Geometry check sheet. Reference: the model listing, model coordinates, mm. A direction names the side the tool comes from. Give positions to 0.01 mm unless a question says otherwise; leave off trailing zeros. Write each loop counter-clockwise with the first axis right and the second up, starting at its lowest first coordinate (ties: lowest second). Pieces come first, ordered by that corner, then holes. Notation, with made-up numbers: (-5.5, 39) - (51.5, 39) arc R25 ccw to (51.5, 72) - close; hole circle Ø8 at (16, 20). An arc over 180 degrees is marked (long way). Use a Markdown table: item, result.
```python
from build123d import *

# Parameters (mm, degrees)
F0_R     = 14.5472790553
F1_DEPTH = 3.175
F2_DEPTH = 5.715


with BuildPart() as f1:
    # F0 (on Top) → F1 (new body)
    with BuildSketch(Plane.XY):
        with BuildLine():
            add(Edge.make_bspline(
                [(-17.3302307441, -18.9114744135), (-12.7840517895, -39.3035737815), (-3.2940015008, -39.2257868182)],
                knots=[5.1919648614, 5.1919648614, 5.1919648614, 6.2831853072, 6.2831853072, 6.2831853072], degree=2, weights=[1, 0.854810781, 1]))
            add(Edge.make_bspline(
                [(-3.2940015008, -39.2257868182), (6.123923112, -39.1485910465), (10.3601545856, -18.9114744135)],
                knots=[0, 0, 0, 1.0844638725, 1.0844638725, 1.0844638725], degree=2, weights=[1, 0.8565590272, 1]))
            add(Edge.make_bspline(
                [(10.3601545856, -18.9114744135), (12.1044870422, -10.5785351982), (12.0273641605, -1.1695031996)],
                knots=[1.0844638725, 1.0844638725, 1.0844638725, 1.5707963268, 1.5707963268, 1.5707963268], degree=2, weights=[1, 0.9705804868, 1]))
            add(Edge.make_bspline(
                [(12.0273641605, -1.1695031996), (11.88861373, 15.7581220548), (6.6027932897, 27.0196823223)],
                knots=[1.5707963268, 1.5707963268, 1.5707963268, 2.4103546369, 2.4103546369, 2.4103546369], degree=2, weights=[1, 0.9131789699, 1]))
            ThreePointArc((6.6027932897, 27.0196823223), (-3.7977289586, 22.4602209118), (-14.2062252861, 27.0014493351))
            add(Edge.make_bspline(
                [(-14.2062252861, 27.0014493351), (-19.3770142282, 15.6392708689), (-19.2371374573, -1.4257685052)],
                knots=[3.8667963971, 3.8667963971, 3.8667963971, 4.7123889804, 4.7123889804, 4.7123889804], degree=2, weights=[1, 0.9119451548, 1]))
            add(Edge.make_bspline(
                [(-19.2371374573, -1.4257685052), (-19.1611285396, -10.6988963006), (-17.3302307441, -18.9114744135)],
                knots=[4.7123889804, 4.7123889804, 4.7123889804, 5.1919648614, 5.1919648614, 5.1919648614], degree=2, weights=[1, 0.9713883601, 1]))
        make_face()
        with Locations((-3.6048866484, -1.2976358524)):
            Circle(F0_R, mode=Mode.SUBTRACT)
    extrude(amount=F1_DEPTH)

    # F0 (on Top) → F2 (join)
    with BuildSketch(Plane.XY):
        with BuildLine():
            add(Edge.make_bspline(
                [(-17.3302307441, -18.9114744135), (-12.7840517895, -39.3035737815), (-3.2940015008, -39.2257868182)],
                knots=[5.1919648614, 5.1919648614, 5.1919648614, 6.2831853072, 6.2831853072, 6.2831853072], degree=2, weights=[1, 0.854810781, 1]))
            add(Edge.make_bspline(
                [(-3.2940015008, -39.2257868182), (6.123923112, -39.1485910465), (10.3601545856, -18.9114744135)],
                knots=[0, 0, 0, 1.0844638725, 1.0844638725, 1.0844638725], degree=2, weights=[1, 0.8565590272, 1]))
            add(Edge.make_bspline(
                [(10.3601545856, -18.9114744135), (12.1044870422, -10.5785351982), (12.0273641605, -1.1695031996)],
                knots=[1.0844638725, 1.0844638725, 1.0844638725, 1.5707963268, 1.5707963268, 1.5707963268], degree=2, weights=[1, 0.9705804868, 1]))
            add(Edge.make_bspline(
                [(12.0273641605, -1.1695031996), (11.88861373, 15.7581220548), (6.6027932897, 27.0196823223)],
                knots=[1.5707963268, 1.5707963268, 1.5707963268, 2.4103546369, 2.4103546369, 2.4103546369], degree=2, weights=[1, 0.9131789699, 1]))
            ThreePointArc((6.6027932897, 27.0196823223), (-3.7977289586, 22.4602209118), (-14.2062252861, 27.0014493351))
            add(Edge.make_bspline(
                [(-14.2062252861, 27.0014493351), (-19.3770142282, 15.6392708689), (-19.2371374573, -1.4257685052)],
                knots=[3.8667963971, 3.8667963971, 3.8667963971, 4.7123889804, 4.7123889804, 4.7123889804], degree=2, weights=[1, 0.9119451548, 1]))
            add(Edge.make_bspline(
                [(-19.2371374573, -1.4257685052), (-19.1611285396, -10.6988963006), (-17.3302307441, -18.9114744135)],
                knots=[4.7123889804, 4.7123889804, 4.7123889804, 5.1919648614, 5.1919648614, 5.1919648614], degree=2, weights=[1, 0.9713883601, 1]))
        make_face()
        with Locations((-3.6048866484, -1.2976358524)):
            Circle(F0_R, mode=Mode.SUBTRACT)
        with BuildLine():
            add(Edge.make_bspline(
                [(10.3601545856, -18.9114744135), (12.1044870422, -10.5785351982), (12.0273641605, -1.1695031996)],
                knots=[1.0844638725, 1.0844638725, 1.0844638725, 1.5707963268, 1.5707963268, 1.5707963268], degree=2, weights=[1, 0.9705804868, 1]))
            Line((10.3601545856, -18.9114744135), (10.3601545856, -45.1457377323))
            Line((10.3601545856, -45.1457377323), (23.0601545856, -45.1457377323))
            Line((23.0601545856, -45.1457377323), (12.0273641605, -1.1695031996))
        make_face()
        with BuildLine():
            Line((-17.3302307441, -45.1457377323), (-17.3302307441, -18.9114744135))
            add(Edge.make_bspline(
                [(-19.2371374573, -1.4257685052), (-19.1611285396, -10.6988963006), (-17.3302307441, -18.9114744135)],
                knots=[4.7123889804, 4.7123889804, 4.7123889804, 5.1919648614, 5.1919648614, 5.1919648614], degree=2, weights=[1, 0.9713883601, 1]))
            Line((-19.2371374573, -1.4257685052), (-30.0302307441, -45.1457377323))
            Line((-30.0302307441, -45.1457377323), (-17.3302307441, -45.1457377323))
        make_face()
        with BuildLine():
            Line((23.0601545856, -45.1457377323), (10.3601545856, -45.1457377323))
            ThreePointArc((10.3601545856, -45.1457377323), (16.7101545856, -53.2856193183), (23.0601545856, -45.1457377323))
        make_face()
        with BuildLine():
            ThreePointArc((-30.0302307441, -45.1457377323), (-23.6802307441, -53.2539903225), (-17.3302307441, -45.1457377323))
            Line((-17.3302307441, -45.1457377323), (-30.0302307441, -45.1457377323))
        make_face()
        with BuildLine():
            ThreePointArc((-14.2062252861, 27.0014493351), (-3.7977289586, 22.4602209118), (6.6027932897, 27.0196823223))
            add(Edge.make_bspline(
                [(6.6027932897, 27.0196823223), (2.1602516195, 36.4846180548), (-3.704532498, 36.6287842303)],
                knots=[2.4103546369, 2.4103546369, 2.4103546369, 3.1280810135, 3.1280810135, 3.1280810135], degree=2, weights=[1, 0.9362966883, 1]))
            ThreePointArc((-3.704532498, 36.6287842303), (-3.8110105262, 36.5248919189), (-3.9157717959, 36.6305151135))
            add(Edge.make_bspline(
                [(-3.9157717959, 36.6305151135), (-9.8462768465, 36.5819046252), (-14.2062252861, 27.0014493351)],
                knots=[3.1415926536, 3.1415926536, 3.1415926536, 3.8667963971, 3.8667963971, 3.8667963971], degree=2, weights=[1, 0.9349770844, 1]))
        make_face()
        with BuildLine():
            add(Edge.make_bspline(
                [(6.6027932897, 27.0196823223), (2.1602516195, 36.4846180548), (-3.704532498, 36.6287842303)],
                knots=[2.4103546369, 2.4103546369, 2.4103546369, 3.1280810135, 3.1280810135, 3.1280810135], degree=2, weights=[1, 0.9362966883, 1]))
            ThreePointArc((6.6027932897, 27.0196823223), (9.387427608, 31.4709155445), (10.3601545856, 36.6305151135))
            ThreePointArc((10.3601545856, 36.6305151135), (9.3748938948, 41.8220601436), (6.55612214, 46.2916691))
            ThreePointArc((6.55612214, 46.2916691), (-3.8101450556, 50.8008147547), (-14.1764122512, 46.2916691))
            ThreePointArc((-14.1764122512, 46.2916691), (-16.9951840059, 41.8220601436), (-17.9804446968, 36.6305151135))
            ThreePointArc((-17.9804446968, 36.6305151135), (-17.0031917826, 31.459353737), (-14.2062252861, 27.0014493351))
            add(Edge.make_bspline(
                [(-3.9157717959, 36.6305151135), (-9.8462768465, 36.5819046252), (-14.2062252861, 27.0014493351)],
                knots=[3.1415926536, 3.1415926536, 3.1415926536, 3.8667963971, 3.8667963971, 3.8667963971], degree=2, weights=[1, 0.9349770844, 1]))
            ThreePointArc((-3.9157717959, 36.6305151135), (-3.8101450556, 36.7361418538), (-3.7045183152, 36.6305151135))
            ThreePointArc((-3.7045183152, 36.6305151135), (-3.704521861, 36.6296496428), (-3.704532498, 36.6287842303))
        make_face()
        with BuildLine():
            ThreePointArc((6.55612214, 46.2916691), (9.3748938948, 41.8220601436), (10.3601545856, 36.6305151135))
            Line((10.3601545856, 36.6305151135), (35.4768335819, 46.2916691))
            Line((35.4768335819, 46.2916691), (35.4768335819, 58.7584972382))
            Line((35.4768335819, 58.7584972382), (20.6948220729, 58.7584972382))
            Line((20.6948220729, 58.7584972382), (6.55612214, 46.2916691))
        make_face()
        with BuildLine():
            Line((-43.2374104858, 46.2916691), (-17.9804446968, 36.6305151135))
            ThreePointArc((-17.9804446968, 36.6305151135), (-16.9951840059, 41.8220601436), (-14.1764122512, 46.2916691))
            Line((-14.1764122512, 46.2916691), (-27.3467302323, 58.7584972382))
            Line((-27.3467302323, 58.7584972382), (-43.2374104858, 58.7584972382))
            Line((-43.2374104858, 58.7584972382), (-43.2374104858, 46.2916691))
        make_face()
    extrude(amount=F2_DEPTH)


solid = f1.part
```
1) Section check A-A on y = -12.5. Record the boundary of the cut face in (x, z) (3 decimals).
Working result:
| item | result |
|---|---|
| outline | (-21.971, 0) - (-12.886, 0) - (-12.886, 5.715) - (-21.971, 5.715) - close; (5.676, 0) - (14.87, 0) - (14.87, 5.715) - (5.676, 5.715) - close |
2) Section check D-D on x = -32. Record the boundary of the cut face in (y, z) (1 decimal).
Working result:
| item | result |
|---|---|
| outline | (42, 0) - (58.8, 0) - (58.8, 5.7) - (42, 5.7) - close |
3) Mould release check, pull along Y, two halves, no side actions. Record for faces 1 (the flat face through (2, 15, 0)), 2 (the flat face through (-24.56, -22.98, 2.82)), 3 (the flat face through (-20.67, 52.44, 2.82)), 4 (the flat face through (22.743, 41.393, 2.817)): pulls with the +Y half, pulls with the -Y half, needs draft (parallel to the pull), parting line crosses it, or undercut.
Working result:
| item | result |
|---|---|
| face 1 | needs draft |
| face 2 | undercut |
| face 3 | pulls with the +Y half |
| face 4 | undercut |
4) Material ranges on L1, parallel to X at y = 47.5, z = 1.55; L2, parallel to X at y = -25, z = 1.3; L3, parallel to X at y = -41.5, z = 2.45, recorded low to high. Write a range as from..to.
Working result:
| item | result |
|---|---|
| L1 | x = -43.24..-15.45, -12.9..5.28, 7.93..35.48 |
| L2 | x = -25.06..-17.33, -15.65..8.76, 10.36..18.01 |
| L3 | x = -29.13..-17.33, 10.36..22.15 |
5) Set-up check for faces 5 (the flat face through (17.621, -23.465, 2.817)), 6 (the cylindrical face through (-17.03, 31.53, 2.82)), 7 (the flat face through (13.72, 52.61, 2.82)): record each of +Z, -Z, +X, -X, +Y, -Y from which the full face is reachable in a straight line by a thin tool's end or side.
Working result:
| item | result |
|---|---|
| face 5 | +Z, -Z, +X |
| face 6 | +Z, -Z, -X |
| face 7 | +Z, -Z, +Y |
6) Depth check by flat-ended pin: P1, Ø2, axis at y = 10.5, z = 3.5, coming from the -X side; P2, Ø3, axis at x = -14, z = 3, coming from the +Y side; P3, Ø2, axis at y = 27, z = 2.5, coming from the +X side. Enter the tip coordinate at first touch or a pass-through.
Working result:
| item | result |
|---|---|
| P1 | stops at x = -18.66 |
| P2 | stops at y = 47.82 |
| P3 | stops at x = 7.43 |
7) Section check C-C on y = -26. Count the separate pieces of the cut face and the enclosed holes in it, then the cut area to 3 significant figures.
Working result:
| item | result |
|---|---|
| separate pieces | 3 |
| enclosed holes | 0 |
| area | 226 mm² |
8) Section check B-B on x = 17. Record the boundary of the cut face in (y, z) (3 decimals), then the cut area to 3 significant figures.
Working result:
| item | result |
|---|---|
| outline | (-53.279, 0) - (-20.99, 0) - (-20.99, 5.715) - (-53.279, 5.715) - close; (39.185, 0) - (55.501, 0) - (55.501, 5.715) - (39.185, 5.715) - close |
| area | 278 mm² |
